Verification items for the finished model (mm, model axes). A direction names the side the tool comes from. Coordinates: 2 decimals unless noted, no trailing zeros. Order: outer loops, then holes, each group sorted by start corner. A loop starts at its lowest first (then second) coordinate and runs counter-clockwise, first axis right, second up. Notation, with made-up numbers: M -12,-18.75 L 35,-18.75 A27 ccw 35,-1.75 Z; hole C 32.5,69.25 d2. An arc over 180 degrees is marked long. Return JSON: item names as keys, results as strings.
```python
from build123d import *

# Parameters (mm, degrees)
SKETCH_2_R          = 1.6
EXTRUDE_1_DEPTH     = 10
SKETCH_3_W          = 8
SKETCH_3_H          = 8
CUT_EXTRUDE_1_DEPTH = 140.947387002
CUT_EXTRUDE_3_DEPTH = 10


with BuildPart() as part:
    # ｽｹｯﾁ2 → ﾎﾞｽ - 押し出し1 (new body)
    with BuildSketch(Plane.XY):
        Polygon((83.071643169, 8.195972832), (-3.936021884, 91.354077293), (-10.845357286, 84.124894469), (77.150331852, 0.022479987), (84.059667254, 7.25166281), align=None)
        with Locations((-3.776098173, 84.28481818)):
            Circle(SKETCH_2_R, mode=Mode.SUBTRACT)
        with Locations((76.990408141, 7.0917391)):
            Circle(SKETCH_2_R, mode=Mode.SUBTRACT)
    extrude(amount=EXTRUDE_1_DEPTH)

    # ｽｹｯﾁ3 → ｶｯﾄ - 押し出し1 (cut, through all)
    with BuildSketch(Plane(origin=(40.308371471, -38.524970914, 0), x_dir=(0, 0, -1), z_dir=(0.7229182823698357, -0.690933540230496, 0))):
        with Locations((-5, 58.32200311)):
            Rectangle(SKETCH_3_W, SKETCH_3_H)
    extrude(amount=-CUT_EXTRUDE_1_DEPTH, mode=Mode.SUBTRACT)

    # ｽｹｯﾁ5 → ｶｯﾄ - 押し出し3 (cut)
    with BuildSketch(Plane(origin=(36.841960381, 38.5474509, 0), x_dir=(0.7229182823698362, -0.6909335402304956, 0), z_dir=(-0.6909335402304956, -0.7229182823698362, 0))):
        with BuildLine():
            ThreePointArc((-11.003582504, 5), (-12.603582504, 6.6), (-14.203582504, 5))
            Line((-14.203582504, 5), (-11.003582504, 5))
        make_face()
        with BuildLine():
            Line((-11.003582504, 5), (-14.203582504, 5))
            ThreePointArc((-14.203582504, 5), (-12.603582504, 3.4), (-11.003582504, 5))
        make_face()
        with BuildLine():
            ThreePointArc((43.996417496, 5), (42.396417496, 6.6), (40.796417496, 5))
            Line((40.796417496, 5), (43.996417496, 5))
        make_face()
        with BuildLine():
            Line((43.996417496, 5), (40.796417496, 5))
            ThreePointArc((40.796417496, 5), (42.396417496, 3.4), (43.996417496, 5))
        make_face()
    extrude(amount=-CUT_EXTRUDE_3_DEPTH, mode=Mode.SUBTRACT)


solid = part.part
```
Q1. Cross-section at A-A, the plane x = 0. Record the boundary of the cut face in (y, z), and give its area (3 significant figures).
Values:
{"outline": "M 73.76,0 L 87.59,0 L 87.59,10 L 73.76,10 Z; hole M 75.14,1 L 86.21,1 L 86.21,9 L 75.14,9 Z", "area": "49.8 mm^2"}
Q2. Tool access check on faces 1 (the face through (-3.98, 85.87, 9.49)), 2 (the face through (34.46, 42.21, 5.06)). Record the directions out of +Z, -Z, +X, -X, +Y, -Y that give a thin tool (end or side, any length) a straight path to the whole face; none if there is none.
Values:
{"face 1": "+Z, -Z", "face 2": "none"}
Q3. Draft check along Z on faces 3 (the face through (-3.98, 85.87, 0.49)), 4 (the face through (33.186, 55.173, 4.519)), 5 (the face through (39.99, 47.99, 5.06)), 6 (the face through (36, 46, 10)). Enter one of: pulls with the +Z half, pulls with the -Z half, needs draft (parallel to the pull), parting line crosses it, or undercut.
Values:
{"face 3": "needs draft", "face 4": "undercut", "face 5": "undercut", "face 6": "pulls with the +Z half"}
Q4. Cross-section at B-B, the plane y = 34.5. Record the boundary of the cut face in (x, z), and give its area (3 significant figures).
Values:
{"outline": "M 41.08,0 L 55.55,0 L 55.55,10 L 41.08,10 Z; hole M 42.52,1 L 54.1,1 L 54.1,9 L 42.52,9 Z", "area": "52.1 mm^2"}
Q5. Material ranges on line 1 along Y through (x, z) = (64, 6.25); line 2 along X through (y, z) = (17, 6.5); line 3 along Y through (x, z) = (18.5, 2.75), recorded low to high.
Values:
{"line 1": "12.59 to 13.97, 25.04 to 26.42", "line 2": "59.39 to 60.83, 72.41 to 73.86", "line 3": "56.08 to 57.46, 68.53 to 69.91"}
Q6. Go/stop test with flat-tipped pins: pin 1 (1.5 mm diameter, centred on y = 53.5, z = 7, fed in from +X); pin 2 (1 mm diameter, centred on x = 74, z = 1.5, fed in from +Y); pin 3 (2 mm diameter, centred on x = 20, z = 6.5, fed in from +Y); pin 4 (3 mm diameter, centred on x = 76.99, y = 7.09, fed in from -Z). Record where each tip stops, or that it passes through.
Values:
{"pin 1": "x = 36.46", "pin 2": "y = 17.34", "pin 3": "y = 69.43", "pin 4": "through"}
